Source: CAD feature listing. Evaluate the final solid. Frame: model axes, mm. A direction names the side the tool comes from. Round coordinates to 2 decimals unless told otherwise and drop trailing zeros.
```python
from build123d import *

# Parameters (mm, degrees)
F1_DEPTH     = 30
F2_R         = 14.99999
F4_DEPTH     = 299.001
F5_T1_DEPTH  = 2e-05
F5_T6_ANGLE  = 163.702935025
F5_T12_ANGLE = 163.702935025
F5_T18_ANGLE = 163.702935025
F5_T24_ANGLE = 163.702935025
F6_SIZE      = 5
F7_R         = 2.5
F8_DEPTH     = 179.001
F9_W         = 20
F9_H         = 20
F11_R        = 2.5
F12_DEPTH    = 20.001
F13_SIZE     = 2.5
F14_W        = 5
F14_H        = 25
F15_DEPTH    = 30
F16_R        = 14.99999
F17_R        = 5
F18_DEPTH    = 7.5
F19_SIZE     = 2.49999


# Not quite as in the source:
# - a fillet or chamfer that OpenCascade refuses, or shapes differently, is made with other operations: its cross-section is extruded or revolved along the edge and cut away or added
# - a fillet or chamfer is up to 0.001 mm smaller than in the source, because OpenCascade refuses the exact size


with BuildPart() as f1:
    # F0 (on Front) → F1 (new body)
    with BuildSketch(Plane.XZ):
        Polygon((-149.5, 0), (0, 0), (149.5, 0), (149.5, 20), (29.5, 20), (29.5, 50), (19.5, 50), (19.5, 20), (0, 20), (-19.5, 20), (-19.5, 50), (-29.5, 50), (-29.5, 20), (-149.5, 20), align=None)
    extrude(amount=F1_DEPTH)

    # F2 (radius 15 in the source; OpenCascade refuses exactly that, so slightly less here)
    f2_edges = [f1.edges().sort_by_distance(p)[0] for p in [
        (-89.5, 0, 20),
        (-89.5, -30, 20),
        (89.5, 0, 20),
        (89.5, -30, 20),
    ]]
    fillet(f2_edges, radius=F2_R)

    # F3 (on face) → F4 (cut, through all)
    with BuildSketch(Plane(origin=(-149.5, 0, 0), x_dir=(0, -1, 0), z_dir=(-1, 0, 0))):
        with BuildLine():
            Line((25, 0), (25, 5))
            ThreePointArc((25, 5), (15, 15), (5, 5))
            Line((5, 5), (5, 0))
            Line((5, 0), (25, 0))
        make_face()
    extrude(amount=-F4_DEPTH, mode=Mode.SUBTRACT)

    # F5: chamfer of 7.5 on 4 edges, made by hand

    # F5_s2 → F5_t1 (join)
    with BuildSketch(Plane.XZ.offset(14.99999)):
        Polygon((-37, 20), (-29.5, 27.5), (-29.5, 20), align=None)
        Polygon((37, 20), (29.5, 27.5), (29.5, 20), align=None)
    extrude(amount=F5_T1_DEPTH)


with BuildPart() as f5_tool4:
    # F5_s5 → F5_t6 (revolve)
    with BuildSketch(Plane(origin=(0, -12.4720838446, -3.6463990318), x_dir=(1, 0, 0), z_dir=(0, -0.9598196681, -0.2806175417))):
        Polygon((-37, -5.9916217418), (-29.5, -13.4916217418), (-29.5, -5.9916217418), align=None)
    revolve(axis=Axis((-29.5, -14.99999, 5.00001), (1, 0, 0)), revolution_arc=F5_T6_ANGLE)

    split(bisect_by=Plane.XZ, keep=Keep.TOP)

    split(bisect_by=Plane.XY, keep=Keep.TOP)


with BuildPart() as f1_1:
    add(f1.part)

    # F5_t3: union F5_tool4
    add(f5_tool4.part)


with BuildPart() as f5_tool10:
    # F5_s11 → F5_t12 (revolve)
    with BuildSketch(Plane(origin=(0, -12.4720838446, -3.6463990318), x_dir=(1, 0, 0), z_dir=(0, -0.9598196681, -0.2806175417))):
        Polygon((29.5, -13.4916217418), (37, -5.9916217418), (29.5, -5.9916217418), align=None)
    revolve(axis=Axis((29.5, -14.99999, 5.00001), (1, 0, 0)), revolution_arc=F5_T12_ANGLE)

    split(bisect_by=Plane.XZ, keep=Keep.TOP)

    split(bisect_by=Plane.XY, keep=Keep.TOP)


with BuildPart() as f1_2:
    add(f1_1.part)

    # F5_t9: union F5_tool10
    add(f5_tool10.part)


with BuildPart() as f5_tool16:
    # F5_s17 → F5_t18 (revolve)
    with BuildSketch(Plane.XZ.offset(15.00001)):
        Polygon((37, 20), (29.5, 27.5), (29.5, 20), align=None)
    revolve(axis=Axis((29.5, -15.00001, 5.00001), (1, 0, 0)), revolution_arc=F5_T18_ANGLE)

    split(bisect_by=Plane.XY, keep=Keep.TOP)

    split(bisect_by=Plane.XZ.offset(30), keep=Keep.BOTTOM)


with BuildPart() as f1_3:
    add(f1_2.part)

    # F5_t15: union F5_tool16
    add(f5_tool16.part)


with BuildPart() as f5_tool22:
    # F5_s23 → F5_t24 (revolve)
    with BuildSketch(Plane.XZ.offset(15.00001)):
        Polygon((-37, 20), (-29.5, 27.5), (-29.5, 20), align=None)
    revolve(axis=Axis((-29.5, -15.00001, 5.00001), (1, 0, 0)), revolution_arc=F5_T24_ANGLE)

    split(bisect_by=Plane.XY, keep=Keep.TOP)

    split(bisect_by=Plane.XZ.offset(30), keep=Keep.BOTTOM)


with BuildPart() as f1_4:
    add(f1_3.part)

    # F5_t21: union F5_tool22
    add(f5_tool22.part)

    # F6
    f6_edges = [f1_4.edges().sort_by_distance(p)[0] for p in [
        (-24.5, 0, 50),
        (-24.5, -30, 50),
        (24.5, 0, 50),
        (24.5, -30, 50),
    ]]
    chamfer(f6_edges, length=F6_SIZE)

    # F7 (on face) → F8 (cut, through all)
    with BuildSketch(Plane.YZ.offset(29.5)):
        with Locations((-15, 40)):
            Circle(F7_R)
    extrude(amount=-F8_DEPTH, mode=Mode.SUBTRACT)

    # F9 (on face) → F10 (join, up to the next surface of F1)
    with BuildSketch(Plane(origin=(0, 0, 0), x_dir=(1, 0, 0), z_dir=(0, 0, -1))):
        with Locations((0, 15)):
            Rectangle(F9_W, F9_H)
    extrude(until=Until.NEXT, dir=(0, 0, 1))

    # F11 (on face) → F12 (cut, through all)
    with BuildSketch(Plane.XY.offset(20)):
        with Locations((0, -15)):
            Circle(F11_R)
    extrude(amount=-F12_DEPTH, mode=Mode.SUBTRACT)

    # F13
    f13_edges = [f1_4.edges().sort_by_distance(p)[0] for p in [
        (-29.5, -17.5, 40),
        (29.5, -17.5, 40),
    ]]
    chamfer(f13_edges, length=F13_SIZE)

    # F14 (on face) → F15 (join, through all)
    with BuildSketch(Plane.XZ.offset(30)):
        with Locations((-152, 12.5)):
            Rectangle(F14_W, F14_H)
        with Locations((152, 12.5)):
            Rectangle(F14_W, F14_H)
    extrude(amount=-F15_DEPTH)

    # F16 (radius 15 in the source; OpenCascade refuses exactly that, so slightly less here)
    f16_edges = [f1_4.edges().sort_by_distance(p)[0] for p in [
        (152, 0, 25),
        (152, -30, 25),
        (-152, -30, 25),
        (-152, 0, 25),
    ]]
    fillet(f16_edges, radius=F16_R)

    # F17 (on face) → F18 (cut)
    with BuildSketch(Plane(origin=(0, 0, 0), x_dir=(1, 0, 0), z_dir=(0, 0, -1))):
        with Locations((0, 15)):
            Circle(F17_R)
    extrude(amount=-F18_DEPTH, mode=Mode.SUBTRACT)

    # F19 (size 2.5 in the source; OpenCascade refuses exactly that, so slightly less here)
    f19_edges = [f1_4.edges().sort_by_distance(p)[0] for p in [
        (-2.5, -15, 7.5),
    ]]
    chamfer(f19_edges, length=F19_SIZE)


solid = f1_4.part
```
1. Access query for faces 4 (the face through (79, -5, 3)), 5 (the face through (92.46, -4.51, 15.72)), 6 (the face through (25, -2, 47)). Directions: +Z, -Z, +X, -X, +Y, -Y. A direction counts if a zero-diameter tool reaches every point of the face in a straight line with its end or side. Return the directions, or none.
2. Pull-direction query (X, two-part tool) for faces 1 (the face through (-94.04, -25.49, 15.72)), 2 (the face through (-24, -28, 47)), 3 (the face through (-29.5, -11, 36)); classes: released by +X, released by -X, zero draft, split by the parting line, or undercut.
3. Line query: line 1 along X through (y, z) = (-20.5, 10); line 2 along X through (y, z) = (-24.5, 33); line 3 along Y through (x, z) = (0, 17). Output: solid intervals per line, ascending.
4. First-contact query: pin 1 (8.5 mm diameter, centred on y = -12, z = 41.5, fed in from +X); pin 2 (9 mm diameter, centred on y = -16.5, z = 41.5, fed in from -X); pin 3 (10 mm diameter, centred on y = -4.5, z = 27.5, fed in from +X). Flat tips, straight axial feed; report the tip coordinate or a pass-through.
Result:
1. face 4: -Z
1. face 5: +Z, +Y
1. face 6: +Z, +X, -X, +Y
2. face 1: undercut
2. face 2: zero draft
2. face 3: released by -X
3. line 1: x = -154.5 to -149.5, -10 to 10, 149.5 to 154.5
3. line 2: x = -29.5 to -19.5, 19.5 to 29.5
3. line 3: y = -30 to -17.5, -12.5 to 0
4. pin 1: stops at x = 29.5
4. pin 2: stops at x = -29.5
4. pin 3: stops at x = 32.17
